Could you check a few things on this model? Use its own coordinates, in mm. A direction names the side the tool comes from. Give positions to 0.01 mm unless a question says otherwise; leave off trailing zeros. Write item = value, one per line. Start each with the question number.
1) I'm going to push flat-ended pins straight in: pin 1 Ø3 at (x, z) = (-0.5, 49.5) entering from -Y; pin 2 Ø2.5 at (x, y) = (0.5, -0.5) entering from -Z; pin 3 Ø6 at (x, y) = (7, 4) entering from -Z; pin 4 Ø1 at (x, z) = (-8, 22) entering from +Y. Where does each tip first touch, or does it pass through?
2) If we mould it in two halves opening along X, with no side actions, what happens to faces 3 (the face through (6.944, 5.324, 42.438)), 4 (the face through (0, -1.618, 51)), 5 (the face through (0, 0, 52.578))? For each: +X half, -X half, draft (parallel to the pull), parting line (faces both ways), or undercut.
3) On a 3-axis mill with a long thin cutter (end or side, diameter ignored), from which of +Z, -Z, +X, -X, +Y, -Y can I reach the whole of each face in a straight line? I mean faces 1 (the face through (1.607, 7.235, 15.954)), 2 (the face through (0, -9, 32.578)). Say none if no direction works.
4) I need wall thicknesses on probe 1 along Y at (x, z) = (0, 45.5); probe 2 along Y at (x, z) = (-2.25, 14.5). Which ranges of each line are inside material? Lowest first, please. Write a range as from..to.
from build123d import *

# Parameters (mm, degrees)
SKETCH3_W           = 13.167666735
SKETCH3_H           = 3.048361989
BOSS_EXTRUDE7_DEPTH = 4


with BuildPart() as part:
    # Sketch1 → Revolve1 (revolve)
    with BuildSketch(Plane(origin=(0, 0, 0), x_dir=(1, 0, 0), z_dir=(0, 1, 0))):
        with BuildLine():
            Line((0, 11.422413793), (0, 8.922413793))
            Line((0, 8.922413793), (-6.034260666, -1.943584812))
            Line((-6.034260666, -1.943584812), (-8.75, -29.577586207))
            Line((-8.75, -29.577586207), (-5.75, -29.577586207))
            Line((-5.75, -29.577586207), (-5.75, -52.577586207))
            Line((-5.75, -52.577586207), (-8.75, -52.577586207))
            Line((-8.75, -52.577586207), (-8.75, -32.577586207))
            Line((-8.75, -32.577586207), (-11.75, -32.577586207))
            add(Edge.make_bspline(
                [(0, 11.422413793), (-1.278423588, 11.417026245), (-3.873144244, 9.558695327), (-5.944786969, 5.627242402), (-7.710873625, 0.905910608), (-8.885618359, -3.570284013), (-9.891395845, -8.594561629), (-10.670483225, -13.791762741), (-11.219012774, -19.122009095), (-11.530237696, -23.790668903), (-11.707521388, -28.093294524), (-11.749966177, -30.922446964), (-11.75, -32.577586207)],
                knots=[0, 0, 0, 0, 0.077095745, 0.191082865, 0.27602247, 0.396033744, 0.482752955, 0.599802605, 0.727919369, 0.821235279, 0.895416594, 1, 1, 1, 1], degree=3))
        make_face()
    revolve(axis=Axis((0, 0, -11.422413793), (0, 0, 1)))

    # Sketch3 → Boss-Extrude7 (add)
    with BuildSketch(Plane.XY.offset(52.577586207)):
        with Locations((0.047139619, -0.094279236)):
            Rectangle(SKETCH3_W, SKETCH3_H)
    extrude(amount=-BOSS_EXTRUDE7_DEPTH)


solid = part.part
Answer list:
q1.pin_1 = -8.75
q1.pin_2 = -11.42
q1.pin_3 = -7.17
q1.pin_4 = 8.59
q2.face_3 = parting line
q2.face_4 = undercut
q2.face_5 = draft
q3.face_1 = none
q3.face_2 = +Z
q4.probe_1 = -8.75..-5.75, 5.75..8.75
q4.probe_2 = -10.47..-6.91, 6.91..10.47
